Design review of the part built by this model. Coordinates are the model's own, in mm. Face numbers are marked on the shaded views. A direction names the side the tool comes from. Coordinates: 2 decimals unless noted, no trailing zeros. Order: outer loops, then holes, each group sorted by start corner. A loop starts at its lowest first (then second) coordinate and runs counter-clockwise, first axis right, second up. Notation, with made-up numbers: M 50.5,-38.75 L 70.5,-38.75 A14 cw 70.5,-13.75 Z; hole C 0.25,-6.5 d10. An arc over 180 degrees is marked long. Use CSV: the item, a comma, the result in double quotes.
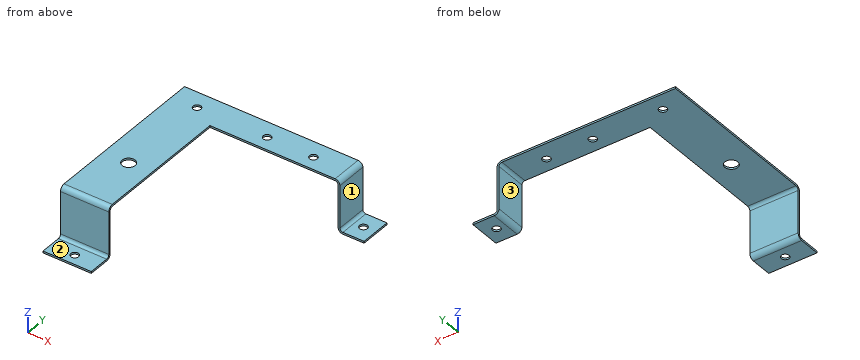
```python
from build123d import *

# Parameters (mm, degrees)
BASE_FLANGE1_DEPTH           = 1
EDGE_FLANGE1_STRIP_W         = 7.2
EDGE_FLANGE1_STRIP_H         = 1
EDGE_FLANGE1_STRIP_CUT_DEPTH = 17
EDGE_FLANGE1_DEPTH           = 17
EDGE_FLANGE2_STRIP_W         = 7.2
EDGE_FLANGE2_STRIP_H         = 1
EDGE_FLANGE2_STRIP_CUT_DEPTH = 17
EDGE_FLANGE2_DEPTH           = 17
EDGE_FLANGE3_STRIP_W         = 7.2
EDGE_FLANGE3_STRIP_H         = 1
EDGE_FLANGE3_STRIP_CUT_DEPTH = 26
EDGE_FLANGE3_DEPTH           = 26
EDGE_FLANGE4_STRIP_W         = 7.2
EDGE_FLANGE4_STRIP_H         = 1
EDGE_FLANGE4_STRIP_CUT_DEPTH = 26
EDGE_FLANGE4_DEPTH           = 26
SKETCH18_R                   = 2.1
CUT_EXTRUDE1_DEPTH           = 6
SKETCH19_R                   = 2.1
CUT_EXTRUDE2_DEPTH           = 40
SKETCH20_R                   = 3.5
CUT_EXTRUDE3_DEPTH           = 40


# Sheet-metal steps are written as plain solids
with BuildPart() as part:
    # Sketch1 → Base-Flange1 (new body)
    with BuildSketch(Plane.XY):
        Polygon((0, 0), (0, 17), (-96, 17), (-96, -75), (-70, -75), (-70, 0), align=None)
    extrude(amount=-BASE_FLANGE1_DEPTH)

    # Edge-Flange1 strip (across the edge) → Edge-Flange1 strip cut (cut)
    with BuildSketch(Plane(origin=(0, 17, -1), x_dir=(-1, 0, 0), z_dir=(0, -1, 0))):
        with Locations((-1, -0.5)):
            Rectangle(EDGE_FLANGE1_STRIP_W, EDGE_FLANGE1_STRIP_H)
    extrude(amount=EDGE_FLANGE1_STRIP_CUT_DEPTH, mode=Mode.SUBTRACT)

    # Edge-Flange1 section (across the edge) → Edge-Flange1 (add)
    with BuildSketch(Plane(origin=(0, 17, -1), x_dir=(-1, 0, 0), z_dir=(0, -1, 0))):
        with BuildLine():
            Line((0, 1.6), (0, 27))
            Line((0, 27), (1, 27))
            Line((1, 27), (1, 1.6))
            ThreePointArc((1, 1.6), (1.46862915, 0.46862915), (2.6, 0))
            Line((2.6, 0), (2.6, -1))
            ThreePointArc((2.6, -1), (0.761522369, -0.238477631), (0, 1.6))
        make_face()
    extrude(amount=EDGE_FLANGE1_DEPTH)

    # Edge-Flange2 strip (across the edge) → Edge-Flange2 strip cut (cut)
    with BuildSketch(Plane(origin=(0, 0, -28), x_dir=(0, 0, 1), z_dir=(0, 1, 0))):
        with Locations((-1, -0.5)):
            Rectangle(EDGE_FLANGE2_STRIP_W, EDGE_FLANGE2_STRIP_H)
    extrude(amount=EDGE_FLANGE2_STRIP_CUT_DEPTH, mode=Mode.SUBTRACT)

    # Edge-Flange2 section (across the edge) → Edge-Flange2 (add)
    with BuildSketch(Plane(origin=(0, 0, -28), x_dir=(0, 0, 1), z_dir=(0, 1, 0))):
        with BuildLine():
            Line((0, 1.6), (0, 13))
            Line((0, 13), (1, 13))
            Line((1, 13), (1, 1.6))
            ThreePointArc((1, 1.6), (1.46862915, 0.46862915), (2.6, 0))
            Line((2.6, 0), (2.6, -1))
            ThreePointArc((2.6, -1), (0.761522369, -0.238477631), (0, 1.6))
        make_face()
    extrude(amount=EDGE_FLANGE2_DEPTH)

    # Edge-Flange3 strip (across the edge) → Edge-Flange3 strip cut (cut)
    with BuildSketch(Plane(origin=(-70, -75, -1), x_dir=(0, 1, 0), z_dir=(-1, 0, 0))):
        with Locations((-1, -0.5)):
            Rectangle(EDGE_FLANGE3_STRIP_W, EDGE_FLANGE3_STRIP_H)
    extrude(amount=EDGE_FLANGE3_STRIP_CUT_DEPTH, mode=Mode.SUBTRACT)

    # Edge-Flange3 section (across the edge) → Edge-Flange3 (add)
    with BuildSketch(Plane(origin=(-70, -75, -1), x_dir=(0, 1, 0), z_dir=(-1, 0, 0))):
        with BuildLine():
            Line((0, 1.6), (0, 27))
            Line((0, 27), (1, 27))
            Line((1, 27), (1, 1.6))
            ThreePointArc((1, 1.6), (1.46862915, 0.46862915), (2.6, 0))
            Line((2.6, 0), (2.6, -1))
            ThreePointArc((2.6, -1), (0.761522369, -0.238477631), (0, 1.6))
        make_face()
    extrude(amount=EDGE_FLANGE3_DEPTH)

    # Edge-Flange4 strip (across the edge) → Edge-Flange4 strip cut (cut)
    with BuildSketch(Plane(origin=(-96, -75, -28), x_dir=(0, 0, 1), z_dir=(1, 0, 0))):
        with Locations((-1, -0.5)):
            Rectangle(EDGE_FLANGE4_STRIP_W, EDGE_FLANGE4_STRIP_H)
    extrude(amount=EDGE_FLANGE4_STRIP_CUT_DEPTH, mode=Mode.SUBTRACT)

    # Edge-Flange4 section (across the edge) → Edge-Flange4 (add)
    with BuildSketch(Plane(origin=(-96, -75, -28), x_dir=(0, 0, 1), z_dir=(1, 0, 0))):
        with BuildLine():
            Line((0, 1.6), (0, 13))
            Line((0, 13), (1, 13))
            Line((1, 13), (1, 1.6))
            ThreePointArc((1, 1.6), (1.46862915, 0.46862915), (2.6, 0))
            Line((2.6, 0), (2.6, -1))
            ThreePointArc((2.6, -1), (0.761522369, -0.238477631), (0, 1.6))
        make_face()
    extrude(amount=EDGE_FLANGE4_DEPTH)

    # Sketch18 → Cut-Extrude1 (cut)
    with BuildSketch(Plane.XY.offset(-27)):
        with Locations((6.5, 8.5)):
            Circle(SKETCH18_R)
    extrude(amount=-CUT_EXTRUDE1_DEPTH, mode=Mode.SUBTRACT)

    # Sketch19 → Cut-Extrude2 (cut)
    with BuildSketch(Plane.XY):
        with Locations((-44.672390486, 7.611585351)):
            Circle(SKETCH19_R)
        with Locations((-82.401549953, 7.538197483)):
            Circle(SKETCH19_R)
        with Locations((-83, -82.3)):
            Circle(SKETCH19_R)
        with Locations((-19.687589167, 7.489085351)):
            Circle(SKETCH19_R)
    extrude(amount=-CUT_EXTRUDE2_DEPTH, mode=Mode.SUBTRACT)

    # Sketch20 → Cut-Extrude3 (cut)
    with BuildSketch(Plane.XY):
        with Locations((-82.401549953, -43.198683771)):
            Circle(SKETCH20_R)
    extrude(amount=-CUT_EXTRUDE3_DEPTH, mode=Mode.SUBTRACT)


solid = part.part
```
(1) Add section C-C on x = -74. State the section outline as (y, z) points, and give its area (3 significant figures).
The answers:
outline,"M -88,-28 L -76.6,-28 A2.6 ccw -74,-25.4 L -74,-2.6 A1.6 cw -72.4,-1 L 17,-1 L 17,0 L -72.4,0 A2.6 ccw -75,-2.6 L -75,-25.4 A1.6 cw -76.6,-27 L -88,-27 Z"
area,"130 mm2"
(2) Add section D-D on y = -2.5. State the section outline as (x, z) points, and give its area (3 significant figures).
The answers:
outline,"M -96,-1 L -70,-1 L -70,0 L -96,0 Z"
area,"26.0 mm2"
(3) Wall thickness on probe 1 along Z at (x, y) = (-24, 10); probe 2 along Y at (x, z) = (-0.5, -26.25); probe 3 along Y at (x, z) = (-83, -27.55): over which ranges is each line inside the solid? List them lowest first.
The answers:
probe 1,"z = -1 to 0"
probe 2,"y = 0 to 17"
probe 3,"y = -88 to -84.4, -80.2 to -75.14"
(4) Add section B-B on x = 6.5. State the section outline as (y, z) points.
The answers:
outline,"M 0,-28 L 6.4,-28 L 6.4,-27 L 0,-27 Z; M 10.6,-28 L 17,-28 L 17,-27 L 10.6,-27 Z"
(5) For the marked faces 1, 2 and 3, list the 3-axis set-ups (+Z, -Z, +X, -X, +Y, -Y) from which the entire face can be reached by the end or side of a thin tool; tool diameter is ignored.
The answers:
face 1,"+Z, +X, +Y, -Y"
face 2,"+Z, +X, -X, -Y"
face 3,"-Z, -X, +Y, -Y"
(6) Add section A-A on z = -13. State the section outline as (x, y) points.
The answers:
outline,"M -96,-75 L -70,-75 L -70,-74 L -96,-74 Z; M -1,0 L 0,0 L 0,17 L -1,17 Z"
(7) Clearance check with flat-ended pins moving along their axes: P1, Ø10, axis at y = -4.5, z = -15.5, coming from the -X side; P2, Ø5.5, axis at x = 9, y = 5.5, coming from the +Z side; P3, Ø9, axis at x = -79.5, y = -80, coming from the +Z side. State where each tip first meets the part, or that it passes through.
The answers:
P1,"stops at x = -1"
P2,"stops at z = -27"
P3,"stops at z = -26.56"
